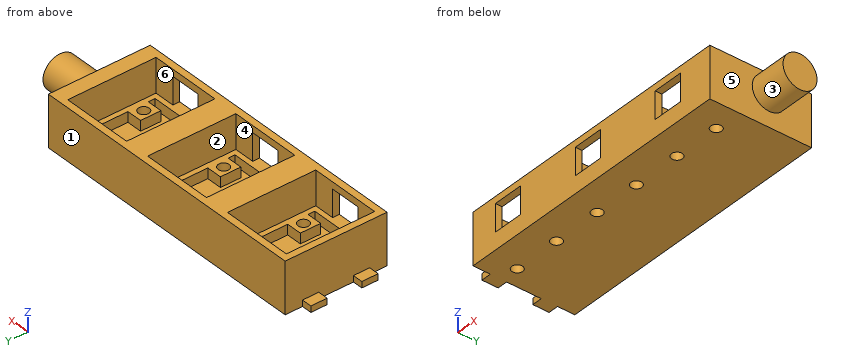
```python
from build123d import *

# Parameters (mm, degrees)
SKETCH_1_W          = 84.5
SKETCH_1_H          = 30
EXTRUDE_1_DEPTH     = 15
SKETCH_2_W          = 21
SKETCH_2_H          = 26
CUT_EXTRUDE_1_DEPTH = 13
SKETCH_3_W          = 21
SKETCH_3_H          = 26
SKETCH_3_W_2        = 18
SKETCH_3_H_2        = 23
EXTRUDE_2_DEPTH     = 3
SKETCH_5_W          = 4.5
SKETCH_5_H          = 6
EXTRUDE_3_DEPTH     = 3
SKETCH_6_R          = 1.6
CUT_EXTRUDE_2_DEPTH = 94.778887913
SKETCH_7_W          = 9
SKETCH_7_H          = 8
CUT_EXTRUDE_3_DEPTH = 90.714734825
SKETCH_13_W         = 1.8
SKETCH_13_H         = 4.8
EXTRUDE_4_DEPTH     = 3
SKETCH_14_R         = 5
EXTRUDE_5_DEPTH     = 11


with BuildPart() as part:
    # ｽｹｯﾁ1 → ﾎﾞｽ - 押し出し1 (new body)
    with BuildSketch(Plane.XY):
        with Locations((-41.65312059, 25.678571429)):
            Rectangle(SKETCH_1_W, SKETCH_1_H)
    extrude(amount=EXTRUDE_1_DEPTH)

    # ｽｹｯﾁ2 → ｶｯﾄ - 押し出し1 (cut)
    with BuildSketch(Plane.XY.offset(15)):
        with Locations((-71.40312059, 25.678571429)):
            Rectangle(SKETCH_2_W, SKETCH_2_H)
        with Locations((-42.90312059, 25.678571429)):
            Rectangle(SKETCH_2_W, SKETCH_2_H)
        with Locations((-14.40312059, 25.678571429)):
            Rectangle(SKETCH_2_W, SKETCH_2_H)
    extrude(amount=-CUT_EXTRUDE_1_DEPTH, mode=Mode.SUBTRACT)

    # ｽｹｯﾁ3 → ﾎﾞｽ - 押し出し2 (add)
    # profile 1 of 3: a face of its own
    with BuildSketch(Plane.XY.offset(2)):
        with Locations((-71.40312059, 25.678571429)):
            Rectangle(SKETCH_3_W, SKETCH_3_H)
        with Locations((-71.40312059, 25.678571429)):
            Rectangle(SKETCH_3_W_2, SKETCH_3_H_2, mode=Mode.SUBTRACT)
    # profile 2 of 3: a face of its own
    with BuildSketch(Plane.XY.offset(2)):
        with Locations((-42.90312059, 25.678571429)):
            Rectangle(SKETCH_3_W, SKETCH_3_H)
        with Locations((-42.90312059, 25.678571429)):
            Rectangle(SKETCH_3_W_2, SKETCH_3_H_2, mode=Mode.SUBTRACT)
    # profile 3 of 3: a face of its own
    with BuildSketch(Plane.XY.offset(2)):
        with Locations((-14.40312059, 25.678571429)):
            Rectangle(SKETCH_3_W, SKETCH_3_H)
        with Locations((-14.40312059, 25.678571429)):
            Rectangle(SKETCH_3_W_2, SKETCH_3_H_2, mode=Mode.SUBTRACT)
    extrude(amount=EXTRUDE_2_DEPTH)

    # ｽｹｯﾁ5 → ﾎﾞｽ - 押し出し3 (add)
    with BuildSketch(Plane.XY.offset(2)):
        with Locations((-64.65312059, 19.178571429)):
            Rectangle(SKETCH_5_W, SKETCH_5_H)
        with Locations((-78.15312059, 19.178571429)):
            Rectangle(SKETCH_5_W, SKETCH_5_H)
        with Locations((-49.65312059, 19.178571429)):
            Rectangle(SKETCH_5_W, SKETCH_5_H)
        with Locations((-36.15312059, 19.178571429)):
            Rectangle(SKETCH_5_W, SKETCH_5_H)
        with Locations((-21.15312059, 19.178571429)):
            Rectangle(SKETCH_5_W, SKETCH_5_H)
        with Locations((-7.65312059, 19.178571429)):
            Rectangle(SKETCH_5_W, SKETCH_5_H)
    extrude(amount=EXTRUDE_3_DEPTH)

    # ｽｹｯﾁ6 → ｶｯﾄ - 押し出し2 (cut, through all)
    with BuildSketch(Plane.XY.offset(5)):
        with Locations((-64.40312059, 19.178571429)):
            Circle(SKETCH_6_R)
        with Locations((-78.40312059, 19.178571429)):
            Circle(SKETCH_6_R)
        with Locations((-49.90312059, 19.178571429)):
            Circle(SKETCH_6_R)
        with Locations((-35.90312059, 19.178571429)):
            Circle(SKETCH_6_R)
        with Locations((-21.40312059, 19.178571429)):
            Circle(SKETCH_6_R)
        with Locations((-7.40312059, 19.178571429)):
            Circle(SKETCH_6_R)
    extrude(amount=-CUT_EXTRUDE_2_DEPTH, mode=Mode.SUBTRACT)

    # ｽｹｯﾁ7 → ｶｯﾄ - 押し出し3 (cut, through all)
    with BuildSketch(Plane(origin=(0, 12.678571429, 0), x_dir=(1, 0, 0), z_dir=(0, 1, 0))):
        with Locations((-71.40312059, -9)):
            Rectangle(SKETCH_7_W, SKETCH_7_H)
        with Locations((-42.90312059, -9)):
            Rectangle(SKETCH_7_W, SKETCH_7_H)
        with Locations((-14.40312059, -9)):
            Rectangle(SKETCH_7_W, SKETCH_7_H)
    extrude(amount=-CUT_EXTRUDE_3_DEPTH, mode=Mode.SUBTRACT)

    # ｽｹｯﾁ13 → ﾎﾞｽ - 押し出し4 (add)
    with BuildSketch(Plane.ZY.offset(83.90312059)):
        with Locations((0.9, 33.178571429)):
            Rectangle(SKETCH_13_W, SKETCH_13_H)
        with Locations((0.9, 18.178571429)):
            Rectangle(SKETCH_13_W, SKETCH_13_H)
    extrude(amount=EXTRUDE_4_DEPTH)

    # ｽｹｯﾁ14 → ﾎﾞｽ - 押し出し5 (add)
    with BuildSketch(Plane(origin=(0.59687941, 0, 0), x_dir=(0, 0, -1), z_dir=(1, 0, 0))):
        with Locations(Location((-9.5, 28.178571429, 0), (0, 0, 180))):
            Circle(SKETCH_14_R)
    extrude(amount=EXTRUDE_5_DEPTH)


solid = part.part
```
Can you work these out from the model? Positions are in its coordinate system, mm. Face numbers are marked on the shaded views. A direction names the side the tool comes from. Round coordinates to 2 decimals unless told otherwise and drop trailing zeros. One line per item, written item: value. Start each with the question number.
1. For the marked faces 1 and 2, which set-ups out of +Z, -Z, +X, -X, +Y, -Y let a thin tool reach every point of the face, with its end or its side?
2. If we mould it in two halves opening along X, with no side actions, what happens to the marked faces 3, 4, 5 and 6? For each: pulls with the +X half, pulls with the -X half, needs draft (parallel to the pull), parting line crosses it, or undercut.
3. If I drill on probe 1 along X at (y, z) = (30.75, 12); probe 2 along X at (y, z) = (36.75, 10); probe 3 along Y at (x, z) = (-10, 3.75), over which ranges is the centre line in solid material (lowest first)?
4. For pin 1 (1.6 mm diameter, centred on y = 12, z = 10.5, fed in from +X); pin 2 (3 mm diameter, centred on y = 32, z = 10.5, fed in from -X); pin 3 (3.5 mm diameter, centred on x = -7.4, y = 19.18, fed in from +Z), each with a flat end and sliding along its axis, tell me the tip position at first contact or that it passes through.
Calculated:
1. face 1: +Z, -Z, +X, -X, +Y
1. face 2: +Z
2. face 3: needs draft
2. face 4: undercut
2. face 5: pulls with the +X half
2. face 6: undercut
3. probe 1: x = -83.9 to -81.9, -60.9 to -53.4, -32.4 to -24.9, -3.9 to 11.6
3. probe 2: x = -83.9 to -81.9, -60.9 to -53.4, -32.4 to -24.9, -3.9 to 0.6
3. probe 3: y = 10.68 to 14.18, 37.18 to 40.68
4. pin 1: stops at x = 0.6
4. pin 2: stops at x = -83.9
4. pin 3: stops at z = 5
